Autodesk Fusion 360 part; units mm, degrees
sketch "MaskV2" plane through (0, 0, 0) normal (0, 0, 1) x (1, 0, 0)
  spline S0 degree 5 poles (-34.2523, 95.3336) (-35.2526, 94.6891) (-37.2409, 93.3658) (-40.1864, 91.2783) (-44.0399, 88.2891) (-48.7276, 84.2113) (-53.2705, 79.8034) (-57.6389, 75.091) (-61.7831, 70.123) (-65.6362, 64.9683) (-69.1279, 59.6986) (-72.1952, 54.3745) (-74.7946, 49.0314) (-76.9151, 43.6626) (-78.5689, 38.2286) (-79.7757, 32.67) (-80.5515, 26.9191) (-80.8926, 20.9126) (-80.7756, 14.597) (-80.1673, 7.9268) (-79.031, 0.8656) (-77.3347, -6.6132) (-75.0591, -14.5257) (-72.1957, -22.8797) (-68.7429, -31.6769) (-64.7038, -40.9156) (-61.0077, -48.6568) (-57.9762, -54.6582) (-55.8403, -58.7457) (-54.7436, -60.8111) knots 0 0 0 0 0 0 0.04 0.08 0.12 0.16 0.2 0.24 0.28 0.32 0.36 0.4 0.44 0.48 0.52 0.56 0.6 0.64 0.68 0.72 0.76 0.8 0.84 0.88 0.92 0.96 1 1 1 1 1 1
  spline S1 degree 5 poles (69.5672, 53.3007) (67.8702, 53.1838) (64.548, 52.9705) (59.7802, 52.7121) (53.8562, 52.4908) (47.173, 52.4234) (41.1946, 52.571) (35.8717, 52.9412) (31.1095, 53.5427) (26.7456, 54.3847) (22.5564, 55.477) (18.3169, 56.8318) (13.8423, 58.4658) (9.0491, 60.4018) (3.9674, 62.668) (-1.3048, 65.2946) (-6.6318, 68.31) (-11.8738, 71.7374) (-16.9248, 75.5895) (-21.7215, 79.8688) (-26.2284, 84.5726) (-29.5909, 88.6705) (-31.975, 91.93) (-33.5034, 94.1853) (-34.2523, 95.3336) knots 0 0 0 0 0 0 0.05 0.1 0.15 0.2 0.25 0.3 0.35 0.4 0.45 0.5 0.55 0.6 0.65 0.7 0.75 0.8 0.85 0.9 0.95 1 1 1 1 1 1
  line L0 (37.7916, 52.8446) -> (43.3291, -44.1745)
  line L1 (-54.7436, -60.8111) -> (75.4385, -38.7276)
  line L2 (69.5672, 53.3007) -> (75.4385, -38.7276)
  circle A0 centre (-17.78, 10.16) radius 9.525
  circle A1 centre (-17.78, 10.16) radius 12.7
  line L3 (-40.1142, -47.6041) -> (19.676, -37.0614) construction
  line L4 (19.676, -37.0614) -> (16.368, -18.3009) construction
  line L5 (16.368, -18.3009) -> (-43.4222, -28.8435) construction
  line L6 (-43.4222, -28.8435) -> (-40.1142, -47.6041) construction
  dimension "d1" = 19.05
  dimension "d2" = 25.4
extrude "Extrude1" add sketch "MaskV2" against normal blind 6.35 contours S0 S1 L0 L1 | A0 | A1
extrude "Extrude2" add sketch "MaskV2" along normal blind 19.05 contours A0
extrude "Extrude3" add sketch "MaskV2" along normal blind 12.7 from surface at 6.35 contours A1
fillet "Fillet1" radius 6.35 1 edges at (-29.6206, 5.5675, 19.05)
chamfer "Chamfer1" distance 3.175 angle 45 1 edges at (-29.6206, 5.5675, 6.35)
fillet "Fillet2" radius 3.81 1 edges at (-29.6206, 14.7525, 9.525)
fillet "Fillet3" radius 3.175 1 edges at (-26.6604, 13.6044, 0)
chamfer "Chamfer3" distance 3.175 angle 45 4 edges at (-5.7072, -52.4928, -6.35) (40.5603, 4.3351, -6.35) (2.2203, 63.5787, -6.35) (-79.1174, 35.4295, -6.35)
Build history of the part. All positions in model axes, mm. A direction names the side the tool comes from. Give positions to 0.01 mm unless a question says otherwise; leave off trailing zeros. Put each result on its own line as item: value.
Item 1: Probe line 1 (Z direction, x = -15, y = -49); line 2 (X direction, y = -37, z = -2); line 3 (X direction, y = 9, z = 9.75). List the from-to ranges inside material, lowest first. Write a range as [from, to].
From the geometry:
line 1: z = [-6.35, 0]
line 2: x = [-66.37, 42.92]
line 3: x = [-30.18, -5.38]
Item 2: 3-axis set-ups, long thin cutter, end or side, ignore diameter. For faces 1 (the flat face through (-6.663, -51.022, -4.785)), 2 (the cylindrical face through (-5.666, 6.345, 11.89)), 3 (the cylindrical face through (-8.98, 13.81, 4.74)): which of +Z, -Z, +X, -X, +Y, -Y reach the whole face in a straight line?
From the geometry:
face 1: -Z, +X, -Y
face 2: +Z
face 3: none
Item 3: Flat gauge pins, fed straight in: pin 1 Ø3 at (x, z) = (-7.5, 8) entering from -Y; pin 2 Ø1.5 at (y, z) = (76.5, -2) entering from -X; pin 3 Ø6 at (x, y) = (-17, 72) entering from +Z. Where does each tip first touch, or does it go through?
From the geometry:
pin 1: stops at y = 2.31
pin 2: stops at x = -56.94
pin 3: stops at z = 0
Item 4: Two-plate mould, pull along Y, no slides. Class faces 4 (the flat face through (-18, 10, 19.05)), 5 (the flat face through (-6.39, -52.61, -1.57)), 6 (the conical face through (-8.57, 13.06, 6.48)), 7 (the flat face through (38.9, 4.9, -4.8)): +Y half, -Y half, draft (parallel to the pull), parting line (faces both ways), or undercut.
From the geometry:
face 4: draft
face 5: -Y half
face 6: parting line
face 7: +Y half
